The listing builds one solid part. Answer for the finished solid, in the listing's coordinates (mm). A direction names the side the tool comes from. Give positions to 0.01 mm unless a question says otherwise; leave off trailing zeros. Write each loop counter-clockwise with the first axis right and the second up, starting at its lowest first coordinate (ties: lowest second). Pieces come first, ordered by that corner, then holes. Notation, with made-up numbers: (28.25, 84.25) - (64.25, 84.25) arc R29 ccw to (64.25, 104.25) - close; hole circle Ø11 at (17.5, 41). An arc over 180 degrees is marked (long way). Write each question's results on one line, items separated by ' | '. Start each with the question number.
Q1. Find the intervals of material crossed by probe 1 along Z at (x, y) = (1, -3.75); probe 2 along Y at (x, z) = (-0.25, 138); probe 3 along Z at (x, y) = (8, 7.5), in increasing order.
Q2. Section B-B (x = -3.25) is taken. Determine the outline of the cut face in (y, z).
Q3. For a pull along Z with two mould halves and no side action, classify faces 1 (the face through (0, 0, -10)), 2 (the face through (0, 12.5, 0)) as pulls with the +Z half, pulls with the -Z half, needs draft (parallel to the pull), parting line crosses it, or undercut.
Q4. Section A-A (y = 0) is taken. Determine the outline of the cut face in (x, z), plus the area to 3 significant figures.
Q5. For faces 3 (the face through (-3.83, -0.175, 249.237)), 4 (the face through (0, -12.5, 0)), determine the directions among +Z, -Z, +X, -X, +Y, -Y from which every point of the face is accessible in a straight line to the end or side of a thin tool.
Q6. Section C-C (z = 48) is taken. Determine the outline of the cut face in (x, y).
Q7. Flat-ended cylindrical pins translate along their axes: pin 1 Ø6 at (x, z) = (4, 133.5) entering from -Y; pin 2 Ø1.5 at (x, y) = (-4.5, -5) entering from +Z; pin 3 Ø3 at (x, z) = (-1, 91) entering from +Y; pin 4 Ø12 at (x, y) = (-3, 7) entering from -Z. Find the tip coordinate at first contact, or state that the pin passes through.
```python
from build123d import *

# Parameters (mm, degrees)
CROQUIS1_R                   = 10
SALIENTE_EXTRUIR1_DEPTH      = 240
SALIENTE_EXTRUIR2_DEPTH      = 12.5
SALIENTE_EXTRUIR2_DEPTH_BACK = 12.5
CROQUIS2_R                   = 10


with BuildPart() as part:
    # Croquis1 → Saliente-Extruir1 (new body)
    with BuildSketch(Plane.XY):
        Circle(CROQUIS1_R)
    extrude(amount=SALIENTE_EXTRUIR1_DEPTH)

    # Croquis2 → Saliente-Extruir2 (add, two sides: drawn at the far end of the back side and taken through both)
    with BuildSketch(Plane(origin=(0, 0, 0), x_dir=(1, 0, 0), z_dir=(0, 1, 0)).offset(-SALIENTE_EXTRUIR2_DEPTH_BACK)):
        with Locations(Location((0, 0, 0), (0, 0, 270))):
            Circle(CROQUIS2_R)
        with Locations(Location((0, -240, 0), (0, 0, 270))):
            Circle(CROQUIS2_R)
    extrude(amount=SALIENTE_EXTRUIR2_DEPTH + SALIENTE_EXTRUIR2_DEPTH_BACK)


solid = part.part
```
Answers below:
1) probe 1: z = -9.95 to 249.95 | probe 2: y = -10 to 10 | probe 3: z = -6 to 6, 234 to 246
2) outline: (-12.5, -9.46) - (12.5, -9.46) - (12.5, 9.46) - (9.46, 9.46) - (9.46, 230.54) - (12.5, 230.54) - (12.5, 249.46) - (-12.5, 249.46) - (-12.5, 230.54) - (-9.46, 230.54) - (-9.46, 9.46) - (-12.5, 9.46) - close
3) face 1: undercut | face 2: needs draft
4) outline: (-10, 0) arc R10 ccw to (10, 0) - (10, 240) arc R10 ccw to (-10, 240) - close | area: 5,110 mm2
5) face 3: none | face 4: +Z, -Z, +X, -X, -Y
6) outline: circle Ø20 at (0, 0)
7) pin 1: stops at y = -9.95 | pin 2: stops at z = 249.27 | pin 3: stops at y = 10 | pin 4: stops at z = -10
